Autodesk Inventor part; units mm, degrees
ref_plane "YZ Plane" through (0, 0, 0) normal (1, 0, 0) x (0, 1, 0)
ref_plane "XZ Plane" through (0, 0, 0) normal (0, 1, 0) x (-1, 0, 0)
ref_plane "XY Plane" through (0, 0, 0) normal (0, 0, 1) x (1, 0, 0)
sketch "Sketch1" plane through (0, 0, 0) normal (0, 1, 0) x (-1, 0, 0)
  line L0 (50, 90) -> (-50, 90)
  line L1 (-50, 90) -> (-50, -90)
  line L2 (-50, -90) -> (50, -90)
  line L3 (50, -90) -> (50, 90)
  point P0 (0, 0)
  dimension "d0" = 100
  dimension "d1" = 180
extrude "Extrusion1" add sketch "Sketch1" along normal blind 19.3
sketch "Sketch2" plane through (0, 19.3, 0) normal (0, 1, 0) x (1, 0, 0)
  line L0 (40.5, -60.5) -> (-40.5, -60.5)
  line L1 (-40.5, -60.5) -> (-40.5, 60.5)
  line L2 (-40.5, 60.5) -> (40.5, 60.5)
  line L3 (40.5, 60.5) -> (40.5, -60.5)
  line L4 (40.5, -60.5) -> (-40.5, 60.5) construction
  line L5 (-40.5, -60.5) -> (40.5, 60.5) construction
  point P0 (0, 0)
  dimension "d4" = 81
  dimension "d5" = 121
extrude "Extrusion2" cut sketch "Sketch2" against normal blind 19.3
fillet "Fillet1" radius 2 4 edges at (-40.5, 9.65, -60.5) (-40.5, 9.65, 60.5) (40.5, 9.65, 60.5) (40.5, 9.65, -60.5)
sketch "Sketch3" plane through (0, 19.3, 0) normal (0, 1, 0) x (1, 0, 0)
  line L0 (-50, 90) -> (-50, -90)
  line L1 (-40.5, -58.5) -> (-40.5, 58.5)
  line L2 (-50, 10.25) -> (-40.5, 10.25)
  line L3 (-40.5, 10.25) -> (-40.5, -10.25)
  line L4 (-40.5, -10.25) -> (-50, -10.25)
  line L5 (-50, -10.25) -> (-50, 10.25)
  line L6 (40.5, 58.5) -> (40.5, -58.5)
  line L7 (50, -90) -> (50, 90)
  line L8 (40.5, 10.25) -> (50, 10.25)
  line L9 (50, 10.25) -> (50, -10.25)
  line L10 (50, -10.25) -> (40.5, -10.25)
  line L11 (40.5, -10.25) -> (40.5, 10.25)
  point P0 (0, 0)
  dimension "d9" = 20.5
extrude "Extrusion3" cut sketch "Sketch3" against normal blind 4.5
properties part number "Cutter-bed"
Read the model definition and answer for the solid it produces. Units are mm, in the model's axes. A direction names the side the tool comes from. Round coordinates to 2 decimals unless told otherwise and drop trailing zeros. Order: outer loops, then holes, each group sorted by start corner. A loop starts at its lowest first (then second) coordinate and runs counter-clockwise, first axis right, second up.
1) A flat-ended cylindrical pin translates along its axis: pin 1 (5 mm diameter, centred on x = 47, z = -3, fed in from +Y). Find the tip coordinate at first contact, or state that the pin passes through.
2) The part is cut by section C-C on x = 33. Write down the section's boundary in (y, z).
3) The part is cut by section B-B on y = 16.5. Write down the section's boundary in (x, z).
4) The mould has two halves that part along Z. Classify faces 4 (the face through (50, 10, 1)), 5 (the face through (45, 14.8, 0)), 6 (the face through (1, 10, -90)): released by +Z, released by -Z, zero draft, split by the parting line, or undercut.
5) Straight lines are drawn through the part: L1, parallel to Z at x = -3, y = 2.5; L2, parallel to X at y = 8.25, z = -3.5; L3, parallel to Z at x = -44.5, y = 17. For each, find the intervals that lie inside material, in ascending order.
6) The part is cut by section A-A on z = 18.5. Write down the section's boundary in (x, y), plus the area to 3 significant figures.
7) For faces 1 (the face through (-45, 14.8, 0)), 2 (the face through (1, 10, 60.5)), 3 (the face through (1, 19.3, -67)), determine the directions among +Z, -Z, +X, -X, +Y, -Y from which every point of the face is accessible in a straight line to the end or side of a thin tool.
Resolved:
1. pin 1: stops at y = 14.8
2. outline: (0, -90) - (19.3, -90) - (19.3, -60.5) - (0, -60.5) - close; (0, 60.5) - (19.3, 60.5) - (19.3, 90) - (0, 90) - close
3. outline: (-50, -90) - (50, -90) - (50, -10.25) - (40.5, -10.25) - (40.5, -58.5) arc R2 cw to (38.5, -60.5) - (-38.5, -60.5) arc R2 cw to (-40.5, -58.5) - (-40.5, -10.25) - (-50, -10.25) - close; (-50, 10.25) - (-40.5, 10.25) - (-40.5, 58.5) arc R2 cw to (-38.5, 60.5) - (38.5, 60.5) arc R2 cw to (40.5, 58.5) - (40.5, 10.25) - (50, 10.25) - (50, 90) - (-50, 90) - close
4. face 4: zero draft
4. face 5: undercut
4. face 6: released by -Z
5. L1: z = -90 to -60.5, 60.5 to 90
5. L2: x = -50 to -40.5, 40.5 to 50
5. L3: z = -90 to -10.25, 10.25 to 90
6. outline: (-50, 0) - (-40.5, 0) - (-40.5, 19.3) - (-50, 19.3) - close; (40.5, 0) - (50, 0) - (50, 19.3) - (40.5, 19.3) - close
6. area: 367 mm2
7. face 1: +X, -X, +Y
7. face 2: +Y, -Y
7. face 3: +Z, -Z, +X, -X, +Y
